Autodesk Inventor part; units mm, degrees
ref_plane "YZ Plane" through (0, 0, 0) normal (1, 0, 0) x (0, 1, 0)
ref_plane "XZ Plane" through (0, 0, 0) normal (0, 1, 0) x (-1, 0, 0)
ref_plane "XY Plane" through (0, 0, 0) normal (0, 0, 1) x (1, 0, 0)
sketch "Sketch1" plane through (0, 0, 0) normal (0, 1, 0) x (-1, 0, 0)
  line L0 (0, 0) -> (25.36, 0)
  line L1 (25.36, 0) -> (25.36, -93.22)
  line L2 (25.36, 0) -> (13.16, 0)
  line L3 (13.16, 0) -> (13.16, -10.27)
  line L4 (13.16, -10.27) -> (13.16, -12.77)
  circle A0 centre (13.16, -12.77) radius 2.5
  line L5 (13.16, -12.77) -> (13.16, -15.27)
  line L6 (13.16, -15.27) -> (13.16, -29.33)
  line L7 (13.16, -29.33) -> (13.16, -31.83)
  circle A1 centre (13.16, -31.83) radius 2.5
  line L8 (13.16, -31.83) -> (13.16, -34.33)
  line L9 (13.16, -34.33) -> (13.16, -48.39)
  line L10 (13.16, -48.39) -> (13.16, -50.89)
  circle A2 centre (13.16, -50.89) radius 2.5
  line L11 (13.16, -50.89) -> (13.16, -53.39)
  line L12 (13.16, -53.39) -> (13.16, -73.79)
  line L13 (13.16, -73.79) -> (13.16, -76.29)
  circle A3 centre (13.16, -76.29) radius 2.5
  line L14 (13.16, -76.29) -> (10.66, -76.29)
  line L15 (10.66, -76.29) -> (-15.82, -76.29)
  line L16 (-15.82, -76.29) -> (-30.095, -76.29)
  circle A4 centre (-30.095, -76.29) radius 14.31
  line L17 (-30.095, -76.29) -> (-30.095, -90.6)
  line L18 (-30.095, -90.6) -> (-30.095, -96.84)
  arc A5 (-46.7119, -64.1995) -> (-28.7399, -96.7953) centre (-30.095, -76.29) ccw
  line L19 (25.36, -93.22) -> (-28.7399, -96.7953)
  line L20 (0, 0) -> (-46.7119, -64.1995)
  dimension "d25" = 28.62
  dimension "d1" = 25.36
  dimension "d2" = 93.22
  dimension "d3" = 12.2
  dimension "d4" = 10.27
  dimension "d5" = 2.5
  dimension "d10" = 14.06
  dimension "d11" = 2.5
  dimension "d12" = 14.06
  dimension "d13" = 2.5
  dimension "d14" = 20.4
  dimension "d15" = 2.5
  dimension "d16" = 26.48
  dimension "d17" = 14.275
  dimension "d26" = 6.24
extrude "Extrusion2" add sketch "Sketch1" along normal blind 3.07 contours L0 L3 A0 L6 A1 L9 A2 L12 A3 L15 A4 L18 A5 L20 | L0 L1 L19 A5 L18 A4 L15 A3 L12 A2 L9 A1 L6 A0 L3
properties part number "Bracket"
Verification items for the finished model (mm, model axes). Coordinates: 2 decimals unless noted, no trailing zeros. Write each loop counter-clockwise with the first axis right and the second up, starting at its lowest first coordinate (ties: lowest second). Pieces come first, ordered by that corner, then holes. Notation, with made-up numbers: M -37,11.25 L 10,11.25 A29 ccw 10,31.25 Z; hole C 24,40 d5. An arc over 180 degrees is marked long. One line per question, with ' | ' between items.
1) Release check for a two-part mould opening along Z. For faces 1 (the face through (-15.47, 1.51, -30.87)), 2 (the face through (5, 3.07, -59)), 3 (the face through (47.93, 1.51, -86.5)) record: +Z half, -Z half, draft (parallel to the pull), parting line (faces both ways), or undercut.
Solutions:
face 1: undercut | face 2: draft | face 3: parting line
2) Sectioned sample at D-D on z = -50.89. Record the cut outline in (x, y), then the cut area to 3 significant figures.
Solutions:
outline: M -25.36,0 L -15.66,0 L -15.66,3.07 L -25.36,3.07 Z; M -10.66,0 L 37.03,0 L 37.03,3.07 L -10.66,3.07 Z | area: 176 mm^2
3) Sectioned sample at B-B on y = 2. Record the cut outline in (x, z) (1 decimal), then the cut area to 3 significant figures.
Solutions:
outline: M -25.4,-93.2 L 28.7,-96.8 A20.6 ccw 46.7,-64.2 L 0,0 L -25.4,0 Z; hole C -13.2,-76.3 d5; hole C -13.2,-50.9 d5; hole C -13.2,-31.8 d5; hole C -13.2,-12.8 d5; hole C 30.1,-76.3 d28.6 | area: 4,680 mm^2
4) Sectioned sample at A-A on z = -76.29. Record the cut outline in (x, y) (3 decimals).
Solutions:
outline: M -25.36,0 L -15.66,0 L -15.66,3.07 L -25.36,3.07 Z; M -10.66,0 L 15.785,0 L 15.785,3.07 L -10.66,3.07 Z; M 44.405,0 L 50.645,0 L 50.645,3.07 L 44.405,3.07 Z
5) Material ranges on L1, parallel to X at y = 1.75, z = -76.29 (3 decimals); L2, parallel to Z at x = -13.16, y = 1.45; L3, parallel to X at y = 2.55, z = -76, recorded low to high.
Solutions:
L1: -25.36 to -15.66, -10.66 to 15.785, 44.405 to 50.645 | L2: -94.03 to -78.79, -73.79 to -53.39, -48.39 to -34.33, -29.33 to -15.27, -10.27 to 0 | L3: -25.36 to -15.64, -10.68 to 15.79, 44.4 to 50.64
6) Sectioned sample at C-C on x = -13. Record the cut outline in (y, z).
Solutions:
outline: M 0,-94.04 L 3.07,-94.04 L 3.07,-78.78 L 0,-78.78 Z; M 0,-73.8 L 3.07,-73.8 L 3.07,-53.38 L 0,-53.38 Z; M 0,-48.4 L 3.07,-48.4 L 3.07,-34.32 L 0,-34.32 Z; M 0,-29.34 L 3.07,-29.34 L 3.07,-15.26 L 0,-15.26 Z; M 0,-10.28 L 3.07,-10.28 L 3.07,0 L 0,0 Z
7) Depth check by flat-ended pin: pin 1 Ø1.5 at (y, z) = (2.5, -61) entering from +X. Enter the tip coordinate at first touch or a pass-through.
Solutions:
pin 1: x = 44.93
